The model under review builds one solid part; all positions refer to its coordinate system, in mm. Face numbers are marked on the shaded views. A direction names the side the tool comes from. Coordinates: 2 decimals unless noted, no trailing zeros. Write each loop counter-clockwise with the first axis right and the second up, starting at its lowest first coordinate (ties: lowest second). Pieces come first, ordered by that corner, then holes.
1) Add section C-C, the plane x = -3. State the section outline as (y, z) points.
2) Add section D-D, the plane z = 3.25. State the section outline as (x, y) points, then the cut area to 3 significant figures.
3) For line 1 (Y direction, x = 0, z = 6.55); line 2 (X direction, y = 0, z = 1.95); line 3 (Y direction, x = 0.75, z = 4), list the stretches that pass through material, from the lowest coordinate up.
4) Machinability: for the marked faces 1, 2, 3 and 4, which of the approach directions +Z, -Z, +X, -X, +Y, -Y give a long, thin tool a straight path to every point of the face, cutting with its end or side? Answer none if there is none.
5) Mouldability with a two-part tool opening along Y and no side actions: class the marked faces 5 and 6 as released by +Y, released by -Y, zero draft, split by the parting line, or undercut.
6) For P1, Ø2, axis at x = -1, y = 0.5, coming from the -Z side; P2, Ø1, axis at x = -3, z = 4.5, coming from the +Y side; P3, Ø4, axis at y = -2.5, z = 1.5, coming from the -X side; P4, Ø1, axis at x = -1, y = 2.5, coming from the -Z side, all flat-tipped, find the tip position at first contact; note any pin that passes through.
7) Add section A-A, the plane x = -0.75. State the section outline as (y, z) points, then the cut area to 3 significant figures.
8) Add section B-B, the plane y = 0. State the section outline as (x, z) points, then the cut area to 3 significant figures.
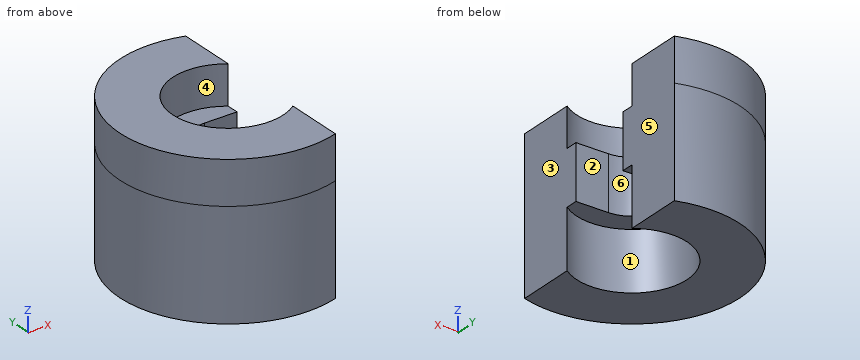
Autodesk Inventor part; units mm, degrees
ref_plane "YZ Plane" through (0, 0, 0) normal (1, 0, 0) x (0, 1, 0)
ref_plane "XZ Plane" through (0, 0, 0) normal (0, 1, 0) x (-1, 0, 0)
ref_plane "XY Plane" through (0, 0, 0) normal (0, 0, 1) x (1, 0, 0)
sketch "Sketch1" plane through (0, 0, 0) normal (0, 0, 1) x (1, 0, 0)
  circle A0 centre (0, 0) radius 5
  dimension "d0" = 10
extrude "Extrusion1" add sketch "Sketch1" along normal blind 5
sketch "Sketch2" plane through (0, 0, 5) normal (0, 0, 1) x (1, 0, 0)
  circle A0 centre (0, 0) radius 5
  arc A1 (0, 1.5) -> (0, -1.5) centre (0, 0) ccw
  line L0 (0, 1.5) -> (4.7697, 1.5)
  line L1 (0, -1.5) -> (4.7697, -1.5)
  arc A2 (4.7697, -1.5) -> (4.7697, 1.5) centre (0, 0) ccw
  dimension "d3" = 3
extrude "Extrusion2" cut sketch "Sketch2" against normal through all contours A0 L1 A1 L0 picked at (1.6667, 0)
sketch "Sketch3" plane through (0, 0, 5) normal (0, 0, 1) x (1, 0, 0)
  arc A0 (0, 1.5) -> (0, -1.5) centre (0, 0) ccw
  line L0 (1.5, 5.5246) -> (5.604, 5.5246)
  line L1 (5.604, 5.5246) -> (5.604, -5.9981)
  line L2 (5.604, -5.9981) -> (1.5, -5.9981)
  line L3 (1.5, -5.9981) -> (1.5, 5.5246)
  dimension "d6" = 1.5
extrude "Extrusion3" cut sketch "Sketch3" against normal through all
sketch "Sketch4" plane through (0, 0, 0) normal (0, 0, -1) x (-1, 0, 0)
  arc A0 (0, -1.5) -> (0, 1.5) centre (0, 0) ccw
  circle A1 centre (0, 0) radius 2.55
  dimension "d9" = 5.1
extrude "Extrusion4" cut sketch "Sketch4" against normal blind 2.7
sketch "Sketch5" plane through (0, 0, 5) normal (0, 0, 1) x (1, 0, 0)
  line L0 (1.5, -4.7697) -> (1.5, -1.5)
  line L1 (1.5, -1.5) -> (0, -1.5)
  arc A0 (0, 1.5) -> (0, -1.5) centre (0, 0) ccw
  line L2 (0, 1.5) -> (1.5, 1.5)
  line L3 (1.5, 1.5) -> (1.5, 4.7697)
  arc A1 (1.5, 4.7697) -> (1.5, -4.7697) centre (0, 0) ccw
extrude "Extrusion5" add sketch "Sketch5" along normal blind 2
sketch "Sketch6" plane through (0, 0, 7) normal (0, 0, 1) x (1, 0, 0)
  arc A0 (1.5, 4.7697) -> (1.5, -4.7697) centre (0, 0) ccw
  circle A1 centre (0, 0) radius 2.55
  dimension "d18" = 5.1
extrude "Extrusion6" cut sketch "Sketch6" against normal blind 1.8
properties part number "Jig_Bearing_Asm_Holder"
Geometry results:
1. outline: (-4, 0) - (4, 0) - (4, 7) - (-4, 7) - close
2. outline: (0, -1.5) arc R1.5 cw to (0, 1.5) - (1.5, 1.5) - (1.5, 4.77) arc R5 ccw (long way) to (1.5, -4.77) - (1.5, -1.5) - close
2. area: 46.0 mm2
3. line 1: y = -5 to -2.55, 2.55 to 5
3. line 2: x = -5 to -2.55
3. line 3: y = -4.94 to -1.5, 1.5 to 4.94
4. face 1: -Z
4. face 2: +Z, -Z, +X
4. face 3: +Z, -Z, +X, +Y, -Y
4. face 4: +Z
5. face 5: zero draft
5. face 6: undercut
6. P1: stops at z = 2.7
6. P2: stops at y = 4.33
6. P3: stops at x = -4.97
6. P4: stops at z = 0
7. outline: (-4.94, 0) - (-2.44, 0) - (-2.44, 2.7) - (-1.3, 2.7) - (-1.3, 5.2) - (-2.44, 5.2) - (-2.44, 7) - (-4.94, 7) - close; (1.3, 2.7) - (2.44, 2.7) - (2.44, 0) - (4.94, 0) - (4.94, 7) - (2.44, 7) - (2.44, 5.2) - (1.3, 5.2) - close
7. area: 40.8 mm2
8. outline: (-5, 0) - (-2.55, 0) - (-2.55, 2.7) - (-1.5, 2.7) - (-1.5, 5.2) - (-2.55, 5.2) - (-2.55, 7) - (-5, 7) - close
8. area: 19.8 mm2
